Input: dimensioned drawing with shaded views. Units: mm. Origin: part minimum x, y, z. A direction names the side the tool comes from. Give positions to 0.01 mm unless a question says otherwise; leave off trailing zeros. Loops run counter-clockwise (first coordinate to the right, second up) from the corner with the lowest first, then second, coordinate; pieces in that order, holes last. Notation, with made-up numbers: (38.25, -30) -> (89.25, -30) arc R29 cw to (89.25, -6) -> close; hole circle Ø2 at (-2.75, -15.75). An arc over 180 degrees is marked (long way). Answer as a JSON object with one key per item and string values.
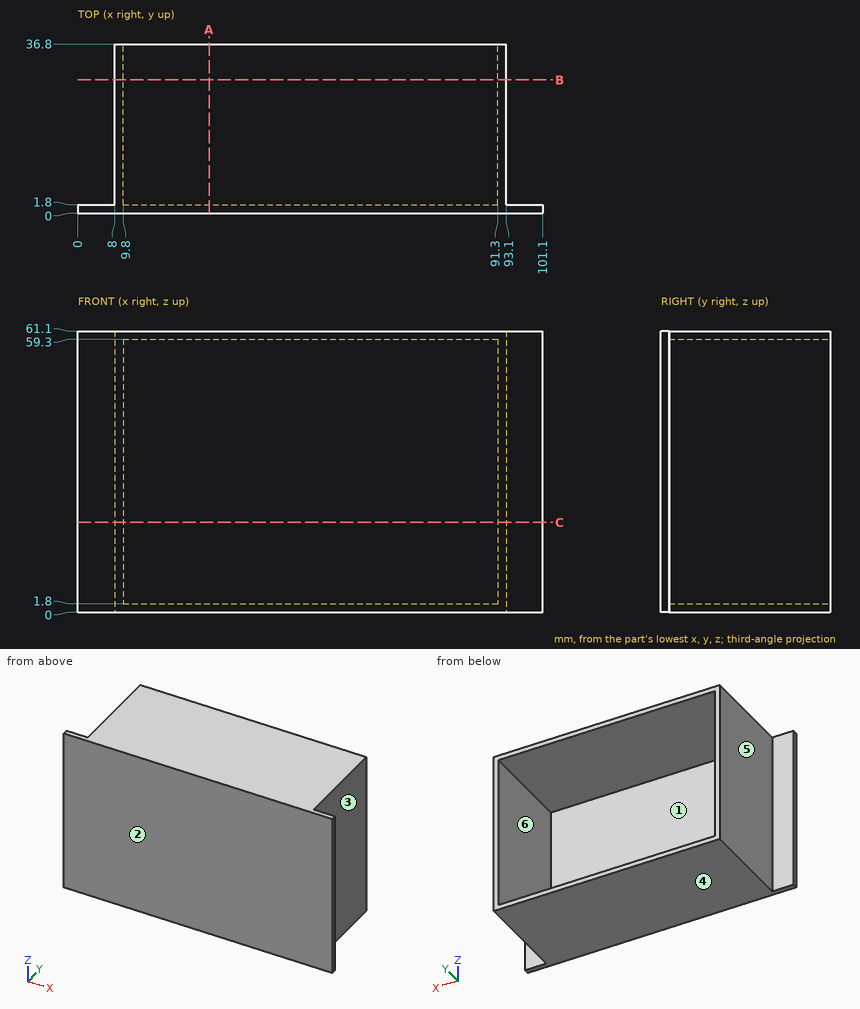
Q1. Draft query along X for the marked faces 1, 2 and 3. Return one class per face: +X half, -X half, draft (parallel to the pull), parting line (faces both ways), or undercut.
Evaluation:
{"face 1": "undercut", "face 2": "draft", "face 3": "+X half"}
Q2. Section C-C, the plane z = 19.5. Return the cut outline in (x, y).
Evaluation:
{"outline": "(0, 0) -> (101.1, 0) -> (101.1, 1.8) -> (93.1, 1.8) -> (93.1, 36.8) -> (91.3, 36.8) -> (91.3, 1.8) -> (9.8, 1.8) -> (9.8, 36.8) -> (8, 36.8) -> (8, 1.8) -> (0, 1.8) -> close"}
Q3. Section B-B, the plane y = 29. Return the cut outline in (x, z), then the cut area to 3 significant figures.
Evaluation:
{"outline": "(8, 0) -> (93.1, 0) -> (93.1, 61.1) -> (8, 61.1) -> close; hole (9.8, 1.8) -> (91.3, 1.8) -> (91.3, 59.3) -> (9.8, 59.3) -> close", "area": "513 mm2"}
Q4. Section A-A, the plane x = 28.5. Return the cut outline in (y, z), then the cut area to 3 significant figures.
Evaluation:
{"outline": "(0, 0) -> (36.8, 0) -> (36.8, 1.8) -> (1.8, 1.8) -> (1.8, 59.3) -> (36.8, 59.3) -> (36.8, 61.1) -> (0, 61.1) -> close", "area": "236 mm2"}
Q5. Access query for the marked faces 4, 5 and 6. Directions: +Z, -Z, +X, -X, +Y, -Y. A direction counts if a zero-diameter tool reaches every point of the face in a straight line with its end or side. Return the directions, or none.
Evaluation:
{"face 4": "-Z, +X, -X, +Y, -Y", "face 5": "+Z, -Z, -X, +Y", "face 6": "+Y"}
Q6. Ray query, line 1 along Z through (x, y) = (84, 35); line 2 along X through (y, z) = (23, 45.5); line 3 along Y through (x, z) = (38, 28). Return the intervals inside material, ascending.
Evaluation:
{"line 1": "z = 0 to 1.8, 59.3 to 61.1", "line 2": "x = 8 to 9.8, 91.3 to 93.1", "line 3": "y = 0 to 1.8"}
Q7. Pin query (flat end, axial travel): pin 1 (6 mm diameter, centred on y = 8, z = 33.5, fed in from +X); pin 2 (6 mm diameter, centred on x = 76, y = 12, fed in from -Z); pin 3 (6 mm diameter, centred on x = 68, z = 20, fed in from +Y); pin 4 (6 mm diameter, centred on y = 20.5, z = 34.5, fed in from -X). Return the tip coordinate at first contact, or that it passes through.
Evaluation:
{"pin 1": "stops at x = 93.1", "pin 2": "stops at z = 0", "pin 3": "stops at y = 1.8", "pin 4": "stops at x = 8"}
